Geometry: final body of the model. Coordinates: model frame, mm. Face numbers are marked on the shaded views. A direction names the side the tool comes from. Coordinates: 2 decimals unless noted, no trailing zeros. Write each loop counter-clockwise with the first axis right and the second up, starting at its lowest first coordinate (ties: lowest second). Pieces come first, ordered by that corner, then holes. Notation, with made-up numbers: M -3,26.5 L 36,26.5 A24 ccw 36,65.5 Z; hole C 56.5,-38 d8. An arc over 180 degrees is marked long. Write item = value, one per line. Start each with the question number.
Item 1: Section D-D on y = -21. Output: boundary loops of the cut face in (x, z), plus the area to 3 significant figures.
Item 2: First-contact query: pin 1 Ø4 at (x, z) = (22, 45.5) entering from +Y; pin 2 Ø3 at (x, y) = (24, -18) entering from +Z. Flat tips, straight axial feed; report the tip coordinate or a pass-through.
Item 3: Section A-A on y = -16.01. Output: boundary loops of the cut face in (x, z), plus the area to 3 significant figures.
Item 4: Reachability of the marked faces 1 and 2 from +Z, -Z, +X, -X, +Y, -Y: full face, straight path, thin tool, end or side. Return the list, or none.
Item 5: Section B-B on x = 24. Output: boundary loops of the cut face in (y, z).
Item 6: Ray query, L1, parallel to Y at x = 34, z = 50; L2, parallel to Z at x = 21, y = -5.5; L3, parallel to Z at x = 8.5, y = -25. Return the intervals inside material, ascending. Write a range as [from, to].
Item 7: Section C-C on z = 45. Output: boundary loops of the cut face in (x, y).
from build123d import *

# Parameters (mm, degrees)
SKETCH1_W              = 43.69375
SKETCH1_H              = 126.6
SKETCH1_R              = 1.4732
BASE_FLANGE1_DEPTH     = 1.6002
SKETCHED_BEND1_DEPTH   = 43.69375
SKETCHED_BEND1_2_DEPTH = 43.69375


# Read off the part's stored shape, not the designer's step: Sketched Bend1
# Sheet-metal steps are written as plain solids
with BuildPart() as part:
    # Sketch1 → Base-Flange1 (new body)
    with BuildSketch(Plane.XY):
        with Locations((21.846875, -63.3)):
            Rectangle(SKETCH1_W, SKETCH1_H)
        with Locations((6.846875, -16.01)):
            Circle(SKETCH1_R, mode=Mode.SUBTRACT)
        with Locations((36.846875, -16.01)):
            Circle(SKETCH1_R, mode=Mode.SUBTRACT)
    extrude(amount=-BASE_FLANGE1_DEPTH)

    # Sketched Bend1 outline → Sketched Bend1 (cut)
    with BuildSketch(Plane.YZ):
        with BuildLine():
            ThreePointArc((-23.640488203, -1.6002), (-25.240688203, -1.171427702), (-26.412115905, 0))
            Line((-26.412115905, 0), (-126.6, 0))
            Line((-126.6, 0), (-126.6, -1.6002))
            Line((-126.6, -1.6002), (-23.640488203, -1.6002))
        make_face()
    extrude(amount=SKETCHED_BEND1_DEPTH, mode=Mode.SUBTRACT)

    # Sketched Bend1 2 outline → Sketched Bend1 2 (add)
    with BuildSketch(Plane.YZ):
        with BuildLine():
            ThreePointArc((-23.640488203, 0), (-24.772000474, 0.468687729), (-25.240688203, 1.6002))
            Line((-25.240688203, 1.6002), (-25.240688203, 101.040688203))
            Line((-25.240688203, 101.040688203), (-26.840888203, 101.040688203))
            Line((-26.840888203, 101.040688203), (-26.840888203, 1.6002))
            ThreePointArc((-26.840888203, 1.6002), (-26.731837217, 0.771875528), (-26.412115905, 0))
            Line((-26.412115905, 0), (-23.640488203, 0))
        make_face()
    extrude(amount=SKETCHED_BEND1_2_DEPTH)


solid = part.part
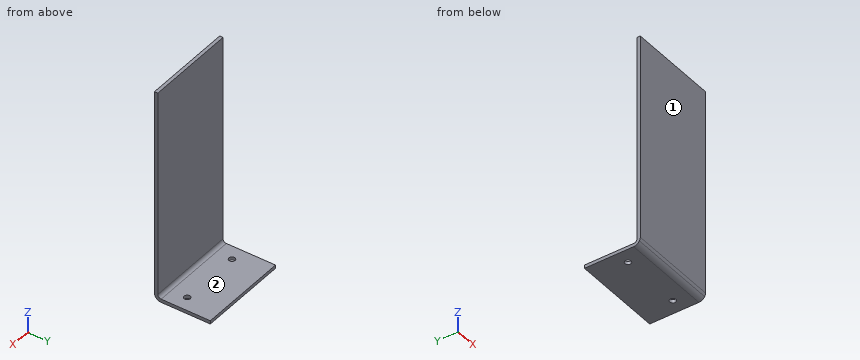
Responses:
q1.outline = M 0,-1.6 L 43.69,-1.6 L 43.69,0 L 0,0 Z
q1.area = 69.9 mm²
q2.pin_1 = -25.24
q2.pin_2 = 0
q3.outline = M 0,-1.6 L 5.37,-1.6 L 5.37,0 L 0,0 Z; M 8.32,-1.6 L 35.37,-1.6 L 35.37,0 L 8.32,0 Z; M 38.32,-1.6 L 43.69,-1.6 L 43.69,0 L 38.32,0 Z
q3.area = 60.5 mm²
q4.face_1 = +Z, -Z, +X, -X, -Y
q4.face_2 = +Z, +X, -X, +Y
q5.outline = M -26.84,1.6 A3.2 ccw -23.64,-1.6 L 0,-1.6 L 0,0 L -23.64,0 A1.6 cw -25.24,1.6 L -25.24,101.04 L -26.84,101.04 Z
q6.L1 = [-26.84, -25.24]
q6.L2 = [-1.6, 0]
q6.L3 = [-1.3, 0.76]
q7.outline = M 0,-26.84 L 43.69,-26.84 L 43.69,-25.24 L 0,-25.24 Z
